```python
from build123d import *

# Parameters (mm, degrees)
F0_R     = 38.1
F1_DEPTH = 12.7
F2_R     = 29.2481
F3_DEPTH = 25.4
F4_SIZE  = 0.635
F6_D     = 5.1054


with BuildPart() as f1:
    # F0 (on Top) → F1 (new body)
    with BuildSketch(Plane.XY):
        Circle(F0_R)
    extrude(amount=F1_DEPTH)

    # F2 (on face) → F3 (join)
    with BuildSketch(Plane.XY.offset(12.7)):
        Circle(F2_R)
    extrude(amount=F3_DEPTH)

    # F4
    f4_edges = [f1.edges().sort_by_distance(p)[0] for p in [
        (-29.2481, 0, 38.1),
        (-38.1, 0, 12.7),
        (-38.1, 0, 0),
    ]]
    chamfer(f4_edges, length=F4_SIZE)

    # F6 (through all)
    with Locations(Plane.XY.offset(38.1)):
        with Locations((0, 0)):
            Hole(F6_D / 2)


solid = f1.part
```
Source: CAD feature listing. Evaluate the final solid. Frame: model axes, mm. A direction names the side the tool comes from. Round coordinates to 2 decimals unless told otherwise and drop trailing zeros. Loops run counter-clockwise (first coordinate to the right, second up) from the corner with the lowest first, then second, coordinate; pieces in that order, holes last.
1. Ray query, L1, parallel to Y at x = 0, z = 21; L2, parallel to Z at x = 28, y = 15; L3, parallel to X at y = -6, z = 19.5. Return the intervals inside material, ascending.
2. Section query C-C on z = 3.5. Output: boundary loops of the cut face in (x, y), and give its area (3 significant figures).
3. Contact query for flat-ended pins moving along their axis: pin 1 (12 mm diameter, centred on y = -18.5, z = 34, fed in from -X); pin 2 (10 mm diameter, centred on x = 3, z = 14, fed in from +Y); pin 3 (4.5 mm diameter, centred on x = 0, y = 0, fed in from +Z); pin 4 (1.5 mm diameter, centred on x = -2, z = 20.5, fed in from -Y). Output: stop coordinate, or through.
4. Section query A-A on x = 0. Output: boundary loops of the cut face in (y, z) (3 decimals).
5. Access query for faces 1 (the flat face through (-1, -8, 0)), 2 (the cylindrical face through (-6.34, -28.553, 24.909)). Directions: +Z, -Z, +X, -X, +Y, -Y. A direction counts if a zero-diameter tool reaches every point of the face in a straight line with its end or side. Return the directions, or none.
6. Section query D-D on z = 30.5. Output: boundary loops of the cut face in (x, y).
Answers below:
1. L1: y = -29.25 to -2.55, 2.55 to 29.25
1. L2: z = 0 to 12.7
1. L3: x = -28.63 to 28.63
2. outline: circle Ø76.2 at (0, 0); hole circle Ø5.11 at (0, 0)
2. area: 4,540 mm2
3. pin 1: stops at x = -26.44
3. pin 2: stops at y = 38.1
3. pin 3: passes through
3. pin 4: stops at y = -29.22
4. outline: (-38.1, 0.635) - (-37.465, 0) - (-2.553, 0) - (-2.553, 38.1) - (-28.613, 38.1) - (-29.248, 37.465) - (-29.248, 12.7) - (-37.465, 12.7) - (-38.1, 12.065) - close; (2.553, 0) - (37.465, 0) - (38.1, 0.635) - (38.1, 12.065) - (37.465, 12.7) - (29.248, 12.7) - (29.248, 37.465) - (28.613, 38.1) - (2.553, 38.1) - close
5. face 1: -Z, +X, -X, +Y, -Y
5. face 2: +Z
6. outline: circle Ø58.5 at (0, 0); hole circle Ø5.11 at (0, 0)
